Geometry check sheet. Reference: the model listing, model coordinates, mm. A direction names the side the tool comes from. Give positions to 0.01 mm unless a question says otherwise; leave off trailing zeros. Loops run counter-clockwise (first coordinate to the right, second up) from the corner with the lowest first, then second, coordinate; pieces in that order, holes last.
1. Cross-section at D-D, the plane z = -12. Record the cut outline in (x, y), plus the area to 3 significant figures.
2. Cross-section at A-A, the plane y = 0. Record the cut outline in (x, z).
3. Release check for a two-part mould opening along Y. For faces 4 (the cylindrical face through (0.56, -12.165, 13.267)), 5 (the flat face through (-127, 0, 0)), 6 (the flat face through (40, 8, 0)) record: +Y half, -Y half, draft (parallel to the pull), parting line (faces both ways), or undercut.
4. Tool access check on faces 1 (the cylindrical face through (82.891, -6.324, -4.032)), 2 (the flat face through (127, 0, 0)), 3 (the cylindrical face through (-148.199, 3.955, 5.158)). Record the directions out of +Z, -Z, +X, -X, +Y, -Y that give a thin tool (end or side, any length) a straight path to the whole face; none if there is none.
5. Material ranges on L1, parallel to Y at x = -155, z = 0; L2, parallel to X at y = 1, z = 15.5; L3, parallel to X at y = 4.5, z = -4, recorded low to high.
6. Cross-section at C-C, the plane x = -88.5. Record the cut outline in (y, z).
7. Go/stop test with flat-tipped pins: pin 1 Ø6.5 at (y, z) = (2, -0.5) entering from -X; pin 2 Ø2 at (x, y) = (42.5, 7.5) entering from -Z; pin 3 Ø12 at (x, y) = (-99.5, 0) entering from +Z; pin 4 Ø17 at (y, z) = (0, 0) entering from -X. Record where each tip stops, or that it passes through.
from build123d import *

# Parameters (mm, degrees)
SKETCH1_W = 80
SKETCH1_H = 10.5


with BuildPart() as part:
    # Sketch1 → Revolve1 (revolve)
    with BuildSketch(Plane.XY, mode=Mode.PRIVATE) as revolve1_sk:
        with Locations((0, 12.75)):
            Rectangle(SKETCH1_W, SKETCH1_H)
        Polygon((-170, 6.5), (-127, 6.5), (-127, 0), (127, 0), (127, 7.5), (-170, 7.5), align=None)
    revolve(revolve1_sk.sketch.rotate(Axis((196.356223274, 0, 0), (-1, 0, 0)), 90), axis=Axis((196.356223274, 0, 0), (-1, 0, 0)))


solid = part.part
Result:
1. outline: (-40, -13.42) - (40, -13.42) - (40, 13.42) - (-40, 13.42) - close
1. area: 2,150 mm2
2. outline: (-170, -7.5) - (-40, -7.5) - (-40, -18) - (40, -18) - (40, -7.5) - (127, -7.5) - (127, 7.5) - (40, 7.5) - (40, 18) - (-40, 18) - (-40, 7.5) - (-170, 7.5) - (-170, 6.5) - (-127, 6.5) - (-127, -6.5) - (-170, -6.5) - close
3. face 4: parting line
3. face 5: undercut
3. face 6: draft
4. face 1: +X
4. face 2: +Z, -Z, +X, +Y, -Y
4. face 3: -X
5. L1: y = -7.5 to -6.5, 6.5 to 7.5
5. L2: x = -40 to 40
5. L3: x = -127 to 127
6. outline: circle Ø15 at (0, 0)
7. pin 1: stops at x = -127
7. pin 2: stops at z = -3.74
7. pin 3: stops at z = 7.5
7. pin 4: stops at x = -170
